```python
from build123d import *

# Parameters (mm, degrees)
SKETCH001_W   = 340
SKETCH001_H   = 575
SKETCH001_R   = 10
SKETCH001_R_2 = 37.5
PAD_DEPTH     = 8
FILLET_R      = 10


with BuildPart() as part:
    # Sketch001 → Pad (new body)
    with BuildSketch(Plane.XY):
        Rectangle(SKETCH001_W, SKETCH001_H)
        with Locations((90, -259.5)):
            Circle(SKETCH001_R, mode=Mode.SUBTRACT)
        with Locations((135, -259.5)):
            Circle(SKETCH001_R, mode=Mode.SUBTRACT)
        with Locations((0, -169.5)):
            Circle(SKETCH001_R_2, mode=Mode.SUBTRACT)
        with BuildLine():
            ThreePointArc((-28.356199, -42.426357), (6.438053, -44.868362), (40.916555, -39.592358))
            ThreePointArc((40.916555, -39.592358), (89.311403, -147.778946), (61.085766, -32.671551))
            ThreePointArc((61.085766, -32.671551), (11.986677, 269.543209), (-82.410869, -21.718846))
            ThreePointArc((-82.410869, -21.718846), (-100.968142, -151.06619), (-28.356199, -42.426357))
        make_face(mode=Mode.SUBTRACT)
    extrude(amount=PAD_DEPTH)

    # Fillet
    fillet_edges = [part.edges().sort_by_distance(p)[0] for p in [
        (-82.410869, -21.718846, 4),
        (40.916555, -39.592358, 4),
        (61.085766, -32.671551, 4),
        (-28.356199, -42.426357, 4),
    ]]
    fillet(fillet_edges, radius=FILLET_R)


solid = part.part
```
CAD build for the part. Positions are in the model's coordinates, mm. Round coordinates to 2 decimals unless told otherwise and drop trailing zeros. Loops run counter-clockwise (first coordinate to the right, second up) from the corner with the lowest first, then second, coordinate; pieces in that order, holes last. Notation, with made-up numbers: M -4.75,13 L 44.25,13 A10 cw 44.25,18 Z; hole C -20.5,-23 d10. An arc over 180 degrees is marked long. Use a Markdown table: item, result. Add a question column.
(1) Drill centre lines: line 1 (X direction, y = -91.5, z = 3.75); line 2 (X direction, y = -88.5, z = 6); line 3 (Y direction, x = -27, z = 7.75). Where is each one in solid material? Low to high.
(2) Flat gauge pin, fed straight in: pin 1 (12 mm diameter, centred on x = 135, y = -259.5, fed in from -Z). Where does the tip first touch, or does it go through?
(3) Cut at B-B (y = 112.5). Give the cut face in (x, z).
(4) Cut at C-C (y = -259.5). Give the cut face in (x, z).
(5) Cut at D-D (x = -77). Give the cut face in (y, z), and give its area (3 significant figures).
(6) Pull direction X, two halves, no side cores. Call faces 1 (the face through (-2, -60, 8)), 2 (the face through (80.01, -259.06, 3.94)): +X half, -X half, draft (parallel to the pull), parting line (faces both ways), or undercut.
(7) Cut at A-A (x = 0). Give the cut face in (y, z).
Geometry says:
| question | item | result |
|---|---|---|
| 1 | line 1 | x = -170 to -143.93, -10.07 to 10.5, 129.5 to 170 |
| 1 | line 2 | x = -170 to -144, -10 to 10.58, 129.42 to 170 |
| 1 | line 3 | y = -287.5 to -195.52, -143.48 to -133.1, 267.67 to 287.5 |
| 2 | pin 1 | passes through |
| 3 | outline | M -170,0 L -157.5,0 L -157.5,8 L -170,8 Z; M 157.5,0 L 170,0 L 170,8 L 157.5,8 Z |
| 4 | outline | M -170,0 L 80,0 L 80,8 L -170,8 Z; M 100,0 L 125,0 L 125,8 L 100,8 Z; M 145,0 L 170,0 L 170,8 L 145,8 Z |
| 5 | outline | M -287.5,0 L -155.5,0 L -155.5,8 L -287.5,8 Z; M 249.89,0 L 287.5,0 L 287.5,8 L 249.89,8 Z |
| 5 | area | 1,360 mm² |
| 6 | face 1 | draft |
| 6 | face 2 | undercut |
| 7 | outline | M -287.5,0 L -207,0 L -207,8 L -287.5,8 Z; M -132,0 L -45,0 L -45,8 L -132,8 Z; M 270,0 L 287.5,0 L 287.5,8 L 270,8 Z |
